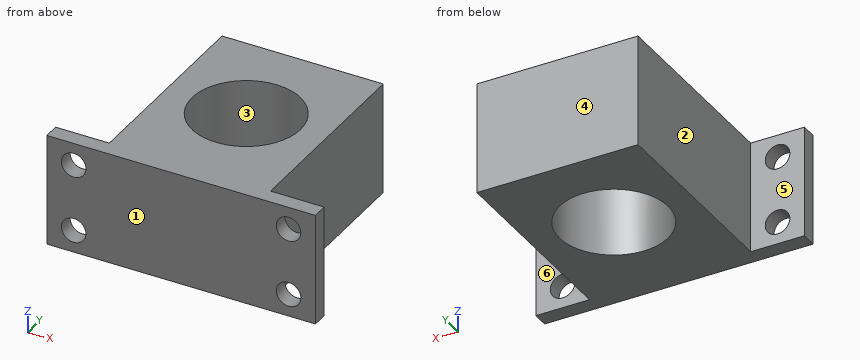
from build123d import *

# Parameters (mm, degrees)
SKETCH3_W           = 18
SKETCH3_H           = 22.5
BRACKETBASE_DEPTH   = 12.5
SKETCH4_R           = 6.05
HOLE_DEPTH          = 13.5
SKETCH5_W           = 30
SKETCH5_H           = 12.5
TABBASE_DEPTH       = 1.75
SKETCH6_R           = 1.375
MOUNTINGHOLES_DEPTH = 2.75


with BuildPart() as part:
    # Sketch3 → bracketBase (new body)
    with BuildSketch(Plane.XY):
        with Locations((9, 11.25)):
            Rectangle(SKETCH3_W, SKETCH3_H)
    extrude(amount=BRACKETBASE_DEPTH)

    # Sketch4 → hole (cut, through all)
    with BuildSketch(Plane.XY.offset(12.5)):
        with Locations((9, 11.25)):
            Circle(SKETCH4_R)
    extrude(amount=-HOLE_DEPTH, mode=Mode.SUBTRACT)

    # Sketch5 → tabBase (add)
    with BuildSketch(Plane.XZ):
        with Locations((9, 6.25)):
            Rectangle(SKETCH5_W, SKETCH5_H)
    extrude(amount=TABBASE_DEPTH)

    # Sketch6 → mountingHoles (cut, through all)
    with BuildSketch(Plane(origin=(0, 0, 0), x_dir=(1, 0, 0), z_dir=(0, 1, 0))):
        with Locations((-3, -2.5)):
            Circle(SKETCH6_R)
        with Locations((-3, -10)):
            Circle(SKETCH6_R)
        with Locations((21, -2.5)):
            Circle(SKETCH6_R)
        with Locations((21, -10)):
            Circle(SKETCH6_R)
    extrude(amount=-MOUNTINGHOLES_DEPTH, mode=Mode.SUBTRACT)


solid = part.part
The listing builds one solid part. Answer for the finished solid, in the listing's coordinates (mm). Face numbers are marked on the shaded views. A direction names the side the tool comes from. Round coordinates to 2 decimals unless told otherwise and drop trailing zeros. Loops run counter-clockwise (first coordinate to the right, second up) from the corner with the lowest first, then second, coordinate; pieces in that order, holes last. Notation, with made-up numbers: M 61,-20.5 L 111,-20.5 A34 ccw 111,14.5 Z; hole C 67,19.25 d6. An arc over 180 degrees is marked long. Return JSON: item names as keys, results as strings.
Q1. Find section A-A, the plane z = 10. Determine the outline of the cut face in (x, y) (3 decimals), plus the area to 3 significant figures.
Results list:
{"outline": "M -6,-1.75 L -4.375,-1.75 L -4.375,0 L -6,0 Z; M -1.625,-1.75 L 19.625,-1.75 L 19.625,0 L 18,0 L 18,22.5 L 0,22.5 L 0,0 L -1.625,0 Z; M 22.375,-1.75 L 24,-1.75 L 24,0 L 22.375,0 Z; hole C 9,11.25 d12.1", "area": "333 mm2"}
Q2. Find section D-D, the plane x = 21. Determine the outline of the cut face in (y, z) (3 decimals), plus the area to 4 significant figures.
Results list:
{"outline": "M -1.75,0 L 0,0 L 0,1.125 L -1.75,1.125 Z; M -1.75,3.875 L 0,3.875 L 0,8.625 L -1.75,8.625 Z; M -1.75,11.375 L 0,11.375 L 0,12.5 L -1.75,12.5 Z", "area": "12.25 mm2"}
Q3. Which of the six approach directions +Z, -Z, +X, -X, +Y, -Y give full straight-line access (tool end or side, diameter ignored) to the marked faces 4, 5 and 6?
Results list:
{"face 4": "+Z, -Z, +X, -X, +Y", "face 5": "+Z, -Z, -X, +Y", "face 6": "+Z, -Z, +X, +Y"}
Q4. Find section B-B, the plane y = 11.25. Determine the outline of the cut face in (x, z).
Results list:
{"outline": "M 0,0 L 2.95,0 L 2.95,12.5 L 0,12.5 Z; M 15.05,0 L 18,0 L 18,12.5 L 15.05,12.5 Z"}
Q5. Find section C-C, the plane x = 9. Determine the outline of the cut face in (y, z).
Results list:
{"outline": "M -1.75,0 L 5.2,0 L 5.2,12.5 L -1.75,12.5 Z; M 17.3,0 L 22.5,0 L 22.5,12.5 L 17.3,12.5 Z"}
Q6. The mould has two halves that part along X. Classify the marked faces 1, 2 and 3: released by +X, released by -X, zero draft, split by the parting line, or undercut.
Results list:
{"face 1": "zero draft", "face 2": "released by -X", "face 3": "undercut"}
Q7. Find the intervals of material crossed by line 1 along X through (y, z) = (-1.35, 2.5) (3 decimals); line 2 along Z through (x, y) = (21, -0.45) (3 decimals); line 3 along Y through (x, z) = (9, 7.5), in increasing order. Write a range as from..to.
Results list:
{"line 1": "x = -6..-4.375, -1.625..19.625, 22.375..24", "line 2": "z = 0..1.125, 3.875..8.625, 11.375..12.5", "line 3": "y = -1.75..5.2, 17.3..22.5"}
Q8. Each of these flat-tipped pins is pushed along its axis until it touches: pin 1 Ø1.5 at (y, z) = (14.5, 10.5) entering from -X; pin 2 Ø2 at (x, z) = (-3, 10) entering from -Y; pin 3 Ø1.8 at (x, z) = (-4, 5.5) entering from +Y. Where does it stop, or does it pass through?
Results list:
{"pin 1": "stops at x = 0", "pin 2": "passes through", "pin 3": "stops at y = 0"}
